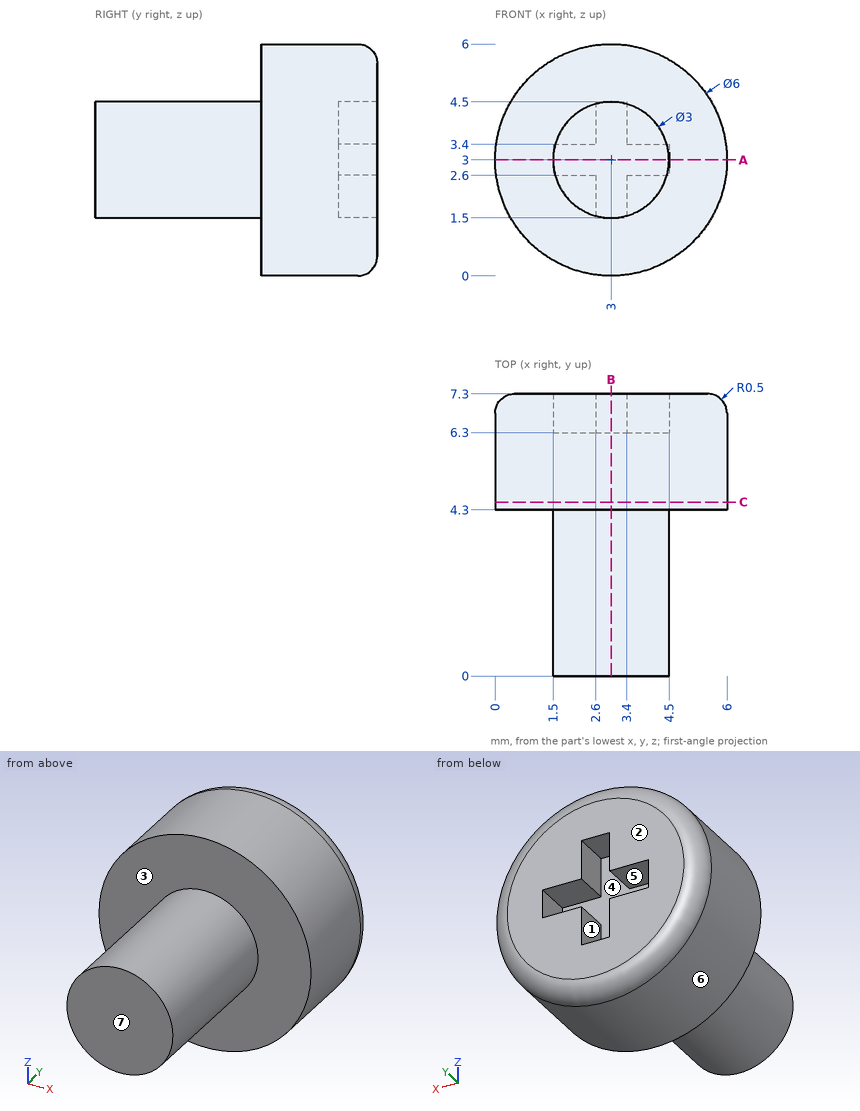
Study the drawing (mm; zero at the part's minimum x, y, z) and answer. A direction names the side the tool comes from. Coordinates: 2 decimals unless noted, no trailing zeros. Write each loop counter-clockwise with the first axis right and the second up, starting at its lowest first coordinate (ties: lowest second). Pieces come first, ordered by that corner, then holes. Notation, with made-up numbers: (-10, 16) - (44, 16) arc R30 cw to (44, 52) - close; hole circle Ø10 at (8, 54.25). An arc over 180 degrees is marked (long way). One line per item, written item: value.
1) Consider line 1 along Y through (x, z) = (2.7, 2.25); line 2 along Y through (x, z) = (4.55, 4.9); line 3 along X through (y, z) = (5.25, 5.55). Determine where each line is inside the solid, lowest interval first. Write a range as from..to.
Geometry check:
line 1: y = 0..6.3
line 2: y = 4.3..7.3
line 3: x = 1.42..4.58
2) Find section C-C (y = 4.5). Give the vertices of the cut face in (x, z).
Geometry check:
outline: circle Ø6 at (3, 3)
3) Each of these flat-tipped pins is pushed along its axis until it touches: pin 1 Ø0.8 at (x, y) = (3.5, 7) entering from +Z; pin 2 Ø1 at (y, z) = (4.5, 2) entering from -X; pin 3 Ø0.6 at (y, z) = (7, 3) entering from +X; pin 4 Ø2 at (x, y) = (2, 1) entering from +Z. Where does it stop, or does it pass through?
Geometry check:
pin 1: stops at z = 6
pin 2: stops at x = 0.04
pin 3: stops at x = 6
pin 4: stops at z = 4.5
4) Find section A-A (z = 3). Give the vertices of the cut face in (x, y), and give its area (3 significant figures).
Geometry check:
outline: (0, 4.3) - (1.5, 4.3) - (1.5, 0) - (4.5, 0) - (4.5, 4.3) - (6, 4.3) - (6, 6.8) arc R0.5 ccw to (5.5, 7.3) - (4.5, 7.3) - (4.5, 6.3) - (1.5, 6.3) - (1.5, 7.3) - (0.5, 7.3) arc R0.5 ccw to (0, 6.8) - close
area: 27.8 mm2
5) For a pull along X with two mould halves and no side action, classify the marked faces 4, 5, 6 and 7 as pulls with the +X half, pulls with the -X half, needs draft (parallel to the pull), parting line crosses it, or undercut.
Geometry check:
face 4: undercut
face 5: undercut
face 6: parting line crosses it
face 7: needs draft
6) A tool of negligible diameter and unlimited length cuts with its end or side. For the marked faces 1, 2 and 3, from which of +Z, -Z, +X, -X, +Y, -Y can it reach the whole face along a straight path? Write none if from no direction.
Geometry check:
face 1: +Y
face 2: +Z, -Z, +X, -X, +Y
face 3: -Y
7) Find section B-B (x = 3). Give the vertices of the cut face in (y, z), and give its area (3 significant figures).
Geometry check:
outline: (0, 1.5) - (4.3, 1.5) - (4.3, 0) - (6.8, 0) arc R0.5 ccw to (7.3, 0.5) - (7.3, 1.5) - (6.3, 1.5) - (6.3, 4.5) - (7.3, 4.5) - (7.3, 5.5) arc R0.5 ccw to (6.8, 6) - (4.3, 6) - (4.3, 4.5) - (0, 4.5) - close
area: 27.8 mm2
